Autodesk Inventor part; units mm, degrees
ref_plane "YZ Plane" through (0, 0, 0) normal (1, 0, 0) x (0, 1, 0)
ref_plane "XZ Plane" through (0, 0, 0) normal (0, 1, 0) x (-1, 0, 0)
ref_plane "XY Plane" through (0, 0, 0) normal (0, 0, 1) x (1, 0, 0)
sketch "Sketch1" plane through (0, 0, 0) normal (0, 0, 1) x (1, 0, 0)
  line L0 (0, 0) -> (49.1491, 34.4146)
  line L1 (0, 0) -> (60, 0) construction
  line L2 (0, 0) -> (45, 0)
  line L3 (45, 0) -> (49.1491, 34.4146)
  line L4 (42.8448, 23.8964) -> (15.858, 5)
  line L5 (15.858, 5) -> (40.5666, 5)
  line L6 (40.5666, 5) -> (42.8448, 23.8964)
  dimension "d0" = 60
  dimension "d1" = 35
  dimension "d2" = 45
  dimension "d3" = 5
extrude "Extrusion1" add sketch "Sketch1" along normal blind 20
ref_plane "Work Plane1" through (0, 0, 10) normal (0, 0, 1) x (1, 0, 0)
sketch "Sketch2" plane through (0, 0, 0) normal (0, -1, 0) x (1, 0, 0)
  point P0 (0, 0)
  point P1 (37.6942, 10.0143)
  point P2 (8.1545, 10.0186)
hole "Hole1" at (37.6942, 0, 10.0143) at (8.1545, 0, 10.0186) direction (0, 1, 0) diameter 3.3 end through all
properties part number "BatteryHolder"
Geometry check sheet. Reference: the model listing, model coordinates, mm. A direction names the side the tool comes from. Coordinates: 2 decimals unless noted, no trailing zeros. Order: outer loops, then holes, each group sorted by start corner. A loop starts at its lowest first (then second) coordinate and runs counter-clockwise, first axis right, second up. Notation, with made-up numbers: (59, 75) - (74, 75) arc R20 ccw to (74, 87) - close; hole circle Ø7 at (25, 88). An arc over 180 degrees is marked (long way). One line per item, written item: value.
(1) Thickness scan on probe 1 along X at (y, z) = (7, 2); probe 2 along X at (y, z) = (13.5, 17); probe 3 along Y at (x, z) = (20.5, 12.25). Record the ranges inside material, lowest first. Write a range as from..to.
Data:
probe 1: x = 10..18.71, 40.81..45.84
probe 2: x = 19.28..28, 41.59..46.63
probe 3: y = 0..5, 8.25..14.35
(2) Sectioned sample at C-C (y = 15). Enter the section's corners in (x, z).
Data:
outline: (21.42, 0) - (30.14, 0) - (30.14, 20) - (21.42, 20) - close; (41.77, 0) - (46.81, 0) - (46.81, 20) - (41.77, 20) - close
(3) Depth check by flat-ended pin: pin 1 Ø3 at (y, z) = (19.5, 11) entering from +X; pin 2 Ø1 at (y, z) = (30.5, 6) entering from -X; pin 3 Ø4 at (y, z) = (9, 5.5) entering from +X; pin 4 Ø4 at (x, y) = (29.5, 11) entering from -Z. Enter the tip coordinate at first touch or a pass-through.
Data:
pin 1: stops at x = 47.53
pin 2: stops at x = 42.84
pin 3: stops at x = 46.33
pin 4: passes through
(4) Sectioned sample at A-A (z = 5.25). Enter the section's corners in (x, y), and give its area (3 significant figures).
Data:
outline: (0, 0) - (45, 0) - (49.15, 34.41) - close; hole (15.86, 5) - (40.57, 5) - (42.84, 23.9) - close
area: 541 mm^2
(5) Sectioned sample at B-B (x = 34). Enter the section's corners in (y, z).
Data:
outline: (0, 0) - (5, 0) - (5, 20) - (0, 20) - close; (17.7, 0) - (23.81, 0) - (23.81, 20) - (17.7, 20) - close
(6) Access from +Z, -Z, +X, -X, +Y, -Y to the whole of each face (thin tool, end or side, straight path). Record for faces 1 (the face through (29.54, 14.58, 9.86)), 2 (the face through (36.3, 2.54, 9.13)).
Data:
face 1: +Z, -Z
face 2: +Y, -Y
(7) Sectioned sample at D-D (z = 11). Enter the section's corners in (x, y).
Data:
outline: (0, 0) - (6.83, 0) - (6.83, 4.78) - close; (9.48, 0) - (36.37, 0) - (36.37, 5) - (15.86, 5) - (36.37, 19.36) - (36.37, 25.47) - (9.48, 6.64) - close; (39.02, 0) - (45, 0) - (49.15, 34.41) - (39.02, 27.32) - (39.02, 21.22) - (42.84, 23.9) - (40.57, 5) - (39.02, 5) - close
(8) Release check for a two-part mould opening along X. For faces 3 (the face through (41.69, 14.32, 9.86)), 4 (the face through (47.046, 16.966, 9.86)), 5 (the face through (28, 15, 0)) record: +X half, -X half, draft (parallel to the pull), parting line (faces both ways), or undercut.
Data:
face 3: undercut
face 4: +X half
face 5: draft
